```python
from build123d import *

# Parameters (mm, degrees)
SKETCH1_R           = 16.15
SKETCH1_R_2         = 11.15
BOSS_EXTRUDE1_DEPTH = 70
BOSS_EXTRUDE2_START = 5
SKETCH2_R           = 16.15
BOSS_EXTRUDE2_DEPTH = 5
CHAMFER1_SIZE       = 5
FILLET1_R           = 2
CHAMFER2_SIZE       = 0.8
SKETCH3_R           = 1.1
CUT_EXTRUDE1_DEPTH  = 10
CIRPATTERN1_COUNT   = 8


with BuildPart() as part:
    # Sketch1 → Boss-Extrude1 (new body)
    with BuildSketch(Plane(origin=(0, 0, 0), x_dir=(1, 0, 0), z_dir=(0, 1, 0))):
        with Locations(Location((0, 0, 0), (0, 0, 270))):
            Circle(SKETCH1_R)
        with Locations(Location((0, 0, 0), (0, 0, 270))):
            Circle(SKETCH1_R_2, mode=Mode.SUBTRACT)
    extrude(amount=BOSS_EXTRUDE1_DEPTH)

    # Sketch2 → Boss-Extrude2 (add)
    with BuildSketch(Plane.XZ.offset(BOSS_EXTRUDE2_START)):
        with Locations(Location((0, 0, 0), (0, 0, 270))):
            Circle(SKETCH2_R)
    extrude(amount=-BOSS_EXTRUDE2_DEPTH)

    # Chamfer1
    chamfer1_edges = [part.edges().sort_by_distance(p)[0] for p in [
        (0, 0, -11.15),
    ]]
    chamfer(chamfer1_edges, length=CHAMFER1_SIZE)

    # Fillet1
    fillet1_edges = [part.edges().sort_by_distance(p)[0] for p in [
        (0, -5, 16.15),
    ]]
    fillet(fillet1_edges, radius=FILLET1_R)

    # Chamfer2
    chamfer2_edges = [part.edges().sort_by_distance(p)[0] for p in [
        (0, 70, -11.15),
    ]]
    chamfer(chamfer2_edges, length=CHAMFER2_SIZE)

    # Sketch3 → Cut-Extrude1 (cut)
    with BuildSketch(Plane(origin=(16.15, 0, 0), x_dir=(0, 0, -1), z_dir=(1, 0, 0))):
        with Locations((0, 64)):
            Circle(SKETCH3_R)
    cut_extrude1 = extrude(amount=-CUT_EXTRUDE1_DEPTH, mode=Mode.SUBTRACT)

    # CirPattern1: Cut-Extrude1 ×8 about axis
    cirpattern1_axis = Axis((0, 69.2, 0), (0, -1, 0))
    for i in range(1, CIRPATTERN1_COUNT):
        add(cut_extrude1.rotate(cirpattern1_axis, i * 360 / CIRPATTERN1_COUNT), mode=Mode.SUBTRACT)


solid = part.part
```
Design review of the part built by this model. Coordinates are the model's own, in mm. A direction names the side the tool comes from. Coordinates: 2 decimals unless noted, no trailing zeros. Order: outer loops, then holes, each group sorted by start corner. A loop starts at its lowest first (then second) coordinate and runs counter-clockwise, first axis right, second up. Notation, with made-up numbers: (21.5, 19) -> (68.5, 19) arc R16 cw to (68.5, 44) -> close; hole circle Ø7 at (-40, 55). An arc over 180 degrees is marked (long way). One line per item, written item: value. Start each with the question number.
Q1. Insertion check: pin 1 Ø2 at (x, y) = (-3.5, 4.5) entering from -Z; pin 2 Ø2 at (y, z) = (21, 12) entering from +X; pin 3 Ø1.5 at (x, y) = (4.5, 39) entering from +Z. Each pin has a flat end and moves straight along its axis. Give the tip position at first contact, or say it passes through.
Q2. Take a section at A-A, the plane x = 0. State the section outline as (y, z) points.
Q3. Take a section at B-B, the plane z = 0. State the section outline as (x, y) points, then the cut area to 3 significant figures.
Q4. Mouldability with a two-part tool opening along Y and no side actions: class faces 1 (the flat face through (12, 70, 2)), 2 (the cylindrical face through (-9.76, 65.09, 9.56)), 3 (the flat face through (0, -5, 0)) as pulls with the +Y half, pulls with the -Y half, needs draft (parallel to the pull), parting line crosses it, or undercut.
Q5. Take a section at C-C, the plane y = 64. Give the number of separate pieces and of enclosed holes in the cut face, then the cut area to 3 significant figures.
Q6. Take a section at D-D, the plane y = 53.5. State the section outline as (x, z) points, then the cut area to 3 significant figures.
Q7. Tool access review of faces 4 (the flat face through (0, 0, 0)), 5 (the cylindrical face through (9.56, 65.09, 9.76)): name each direction out of +Z, -Z, +X, -X, +Y, -Y from which nothing blocks a thin tool from reaching the whole face with its end or side.
Q8. For probe 1 along Y at (x, z) = (-13.85, 0); probe 2 along Z at (x, y) = (12.8, 64); probe 3 along X at (y, z) = (3, -6), list the stretches that pass through material, from the lowest coordinate up.
Values follow:
1. pin 1: stops at z = -15.96
1. pin 2: stops at x = 11.82
1. pin 3: stops at z = 15.71
2. outline: (-5, -14.15) arc R2 ccw to (-3, -16.15) -> (62.9, -16.15) -> (62.9, -11.15) -> (5, -11.15) -> (0, -6.15) -> (0, 6.15) -> (5, 11.15) -> (62.9, 11.15) -> (62.9, 16.15) -> (-3, 16.15) arc R2 ccw to (-5, 14.15) -> close; (65.1, -16.15) -> (70, -16.15) -> (70, -11.95) -> (69.2, -11.15) -> (65.1, -11.15) -> close; (65.1, 11.15) -> (69.2, 11.15) -> (70, 11.95) -> (70, 16.15) -> (65.1, 16.15) -> close
3. outline: (-16.15, -3) arc R2 ccw to (-14.15, -5) -> (14.15, -5) arc R2 ccw to (16.15, -3) -> (16.15, 62.9) -> (11.15, 62.9) -> (11.15, 5) -> (6.15, 0) -> (-6.15, 0) -> (-11.15, 5) -> (-11.15, 62.9) -> (-16.15, 62.9) -> close; (-16.15, 65.1) -> (-11.15, 65.1) -> (-11.15, 69.2) -> (-11.95, 70) -> (-16.15, 70) -> close; (11.15, 65.1) -> (16.15, 65.1) -> (16.15, 70) -> (11.95, 70) -> (11.15, 69.2) -> close
3. area: 862 mm2
4. face 1: pulls with the +Y half
4. face 2: undercut
4. face 3: pulls with the -Y half
5. separate pieces: 8
5. enclosed holes: 0
5. area: 341 mm2
6. outline: circle Ø32.3 at (0, 0); hole circle Ø22.3 at (0, 0)
6. area: 429 mm2
7. face 4: +Y
7. face 5: none
8. probe 1: y = -5 to 62.9, 65.1 to 70
8. probe 2: z = -9.85 to -1.1, 1.1 to 9.85
8. probe 3: x = -14.99 to -6.91, 6.91 to 14.99
